Check sheet for the modelled part. Datum: model origin and axes. Units: mm. Face numbers are marked on the shaded views. A direction names the side the tool comes from. Give positions to 0.01 mm unless a question says otherwise; leave off trailing zeros. Order: outer loops, then holes, each group sorted by start corner. A loop starts at its lowest first (then second) coordinate and runs counter-clockwise, first axis right, second up. Notation, with made-up numbers: M 84,-19 L 108,-19 A14 ccw 108,-6 Z; hole C 37,53.25 d8. An arc over 180 degrees is marked long. Return JSON: item names as keys, results as strings. Group by question number.
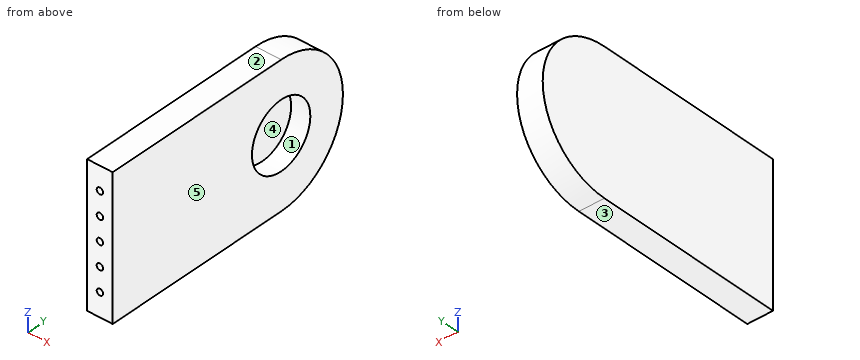
from build123d import *

# Parameters (mm, degrees)
BOSS_EXTRUDE1_DEPTH             = 20
SKETCH3_R                       = 26
CUT_EXTRUDE1_DEPTH              = 15
TAP_DRILL_FOR_M6X1_0_TAP2_D     = 5
TAP_DRILL_FOR_M6X1_0_TAP2_DEPTH = 40
TAP_DRILL_FOR_M6X1_0_TAP2_TIP   = 1.502151548


with BuildPart() as part:
    # Sketch2 → Boss-Extrude1 (new body)
    with BuildSketch(Plane(origin=(0, 0, 0), x_dir=(0, 0, -1), z_dir=(1, 0, 0))):
        with BuildLine():
            Line((55, -75), (55, 75))
            ThreePointArc((55, 75), (0, 20), (-55, 75))
            Line((-55, 75), (-55, -75))
            Line((-55, -75), (55, -75))
        make_face()
        with BuildLine():
            ThreePointArc((-55, 75), (0, 20), (55, 75))
            Line((55, 75), (-55, 75))
        make_face()
        with BuildLine():
            Line((-55, 75), (55, 75))
            ThreePointArc((55, 75), (0, 130), (-55, 75))
        make_face()
    extrude(amount=BOSS_EXTRUDE1_DEPTH)

    # Sketch3 → Cut-Extrude1 (cut)
    with BuildSketch(Plane(origin=(20, 0, 0), x_dir=(0, 0, -1), z_dir=(1, 0, 0))):
        with Locations((0, 75)):
            Circle(SKETCH3_R)
    extrude(amount=-CUT_EXTRUDE1_DEPTH, mode=Mode.SUBTRACT)

    # Tap Drill for M6x1.0 Tap2
    with Locations(Plane(origin=(0, -75, 0), x_dir=(-1, 0, 0), z_dir=(0, -1, 0))):
        with Locations((-10, -36.666666667), (-10, -18.333333333), (-10, 0), (-10, 18.333333333), (-10, 36.666666667)):
            Hole(TAP_DRILL_FOR_M6X1_0_TAP2_D / 2, depth=TAP_DRILL_FOR_M6X1_0_TAP2_DEPTH)
            with Locations((0, 0, -(TAP_DRILL_FOR_M6X1_0_TAP2_DEPTH + TAP_DRILL_FOR_M6X1_0_TAP2_TIP / 2))):  # 118° drill point
                Cone(0, TAP_DRILL_FOR_M6X1_0_TAP2_D / 2, TAP_DRILL_FOR_M6X1_0_TAP2_TIP, mode=Mode.SUBTRACT)


solid = part.part
1) Release check for a two-part mould opening along Z. For the marked faces 3, 4 and 5 record: released by +Z, released by -Z, zero draft, split by the parting line, or undercut.
2) Depth check by flat-ended pin: P1, Ø4, axis at x = 10, z = 18.33, coming from the -Y side; P2, Ø1, axis at y = 64, z = 2.5, coming from the +X side; P3, Ø10, axis at x = 14.5, z = 35, coming from the +Y side. Enter the tip coordinate at first touch or a pass-through.
3) Sectioned sample at D-D on x = 2.5. Record the boundary of the cut face in (y, z), then the cut area to 3 significant figures.
4) Material ranges on line 1 along Z through (x, y) = (10, -53); line 2 along Y through (x, z) = (12.75, 0); line 3 along Y through (x, z) = (13.75, 15.5), recorded low to high.
5) Sectioned sample at C-C on y = 104. Record the boundary of the cut face in (x, z), then the cut area to 3 significant figures.
6) Sectioned sample at A-A on x = 16.75. Record the boundary of the cut face in (y, z).
7) Tool access check on the marked faces 1 and 2. Record the directions out of +Z, -Z, +X, -X, +Y, -Y that give a thin tool (end or side, any length) a straight path to the whole face; none if there is none.
8) Sectioned sample at B-B on z = -23. Record the boundary of the cut face in (x, y).
Reply:
{
 "1": {"face 3": "released by -Z", "face 4": "undercut", "face 5": "zero draft"},
 "2": {"P1": "y = -34.7", "P2": "x = 5", "P3": "y = 121.1"},
 "3": {"outline": "M -75,-55 L 75,-55 A55 ccw 75,55 L -75,55 Z", "area": "21,300 mm^2"},
 "4": {"line 1": "-55 to -39.17, -34.17 to -20.83, -15.83 to -2.5, 2.5 to 15.83, 20.83 to 34.17, 39.17 to 55", "line 2": "-75 to 49, 101 to 130", "line 3": "-75 to 54.13, 95.87 to 127.77"},
 "5": {"outline": "M 0,-46.73 L 20,-46.73 L 20,46.73 L 0,46.73 Z", "area": "1,870 mm^2"},
 "6": {"outline": "M -75,-55 L 75,-55 A55 ccw 75,55 L -75,55 Z; hole C 75,0 d52"},
 "7": {"face 1": "+X", "face 2": "+Z, +X, -X, +Y, -Y"},
 "8": {"outline": "M 0,-75 L 20,-75 L 20,62.88 L 5,62.88 L 5,87.12 L 20,87.12 L 20,124.96 L 0,124.96 Z"}
}
